For this review, take the finished solid that the model builds, in its own axes (mm). A direction names the side the tool comes from. Coordinates: 2 decimals unless noted, no trailing zeros. Loops run counter-clockwise (first coordinate to the right, second up) from the corner with the lowest first, then second, coordinate; pieces in that order, holes last. Notation, with made-up numbers: (-31.5, -39) - (-22.5, -39) arc R22 ccw to (-22.5, -25) - close; hole circle Ø1 at (12, 28). An arc over 180 degrees is marked (long way). One line per item, written item: value. Start each with the question number.
1. Take a section at D-D, the plane x = 16. State the section outline as (y, z) points, and give its area (3 significant figures).
2. Take a section at A-A, the plane y = 0. State the section outline as (x, z) points, and give its area (3 significant figures).
3. Take a section at C-C, the plane z = 0.8. State the section outline as (x, y) points, and give its area (3 significant figures).
4. Insertion check: pin 1 (1.5 mm diameter, centred on y = -10.5, z = 2, fed in from -X); pin 2 (0.6 mm diameter, centred on x = -22, z = 3.5, fed in from -Y); pin 3 (1 mm diameter, centred on y = 17.5, z = 4, fed in from +X). Each pin has a flat end and moves straight along its axis. Give the tip position at first contact, or say it passes through.
5. Take a section at B-B, the plane x = 38.25. State the section outline as (y, z) points.
6. To check wall thickness, follow line 1 (X direction, y = 26, z = 3.1); line 2 (X direction, y = -14.5, z = 2.2); line 3 (Z direction, x = 14, y = 8). State the ranges of each line that lie inside material, in increasing order. Write a range as from..to.
7. For faces 1 (the face through (0, 0, 4)), 2 (the face through (-1, 1, 0)), list the 3-axis set-ups (+Z, -Z, +X, -X, +Y, -Y) from which the entire face can be reached by the end or side of a thin tool; tool diameter is ignored.
```python
from build123d import *

# Parameters (mm, degrees)
F0_R     = 45
F0_R_2   = 1.5
F1_DEPTH = 5
F2_R     = 30
F3_DEPTH = 3
F5_DEPTH = 2


with BuildPart() as f1:
    # F0 (on Top) → F1 (new body)
    with BuildSketch(Plane.XY):
        Circle(F0_R)
        with Locations((-38.25, 0)):
            Circle(F0_R_2, mode=Mode.SUBTRACT)
        with Locations((38.25, 0)):
            Circle(F0_R_2, mode=Mode.SUBTRACT)
    extrude(amount=F1_DEPTH)

    # F2 (on face) → F3 (cut)
    with BuildSketch(Plane.XY.offset(5)):
        Circle(F2_R)
    extrude(amount=-F3_DEPTH, mode=Mode.SUBTRACT)

    # F4 (on face) → F5 (join)
    with BuildSketch(Plane.XY.offset(2)):
        with BuildLine():
            Line((-3.2170990016, 29.8270057836), (-3.2170990016, 2.8556571342))
            Line((-3.2170990016, 2.8556571342), (-29.8637777639, 2.8556571342))
            ThreePointArc((-29.8637777639, 2.8556571342), (-30, 0), (-29.8637777639, -2.8556571342))
            Line((-29.8637777639, -2.8556571342), (-3.2170990016, -2.8556571342))
            Line((-3.2170990016, -2.8556571342), (-3.2170990016, -29.8270057836))
            ThreePointArc((-3.2170990016, -29.8270057836), (0, -30), (3.2170990016, -29.8270057836))
            Line((3.2170990016, -29.8270057836), (3.2170990016, -2.8556571342))
            Line((3.2170990016, -2.8556571342), (29.8637777639, -2.8556571342))
            ThreePointArc((29.8637777639, -2.8556571342), (29.9659250893, -1.4294521823), (30, 0))
            ThreePointArc((30, 0), (29.9659250893, 1.4294521823), (29.8637777639, 2.8556571342))
            Line((29.8637777639, 2.8556571342), (3.2170990016, 2.8556571342))
            Line((3.2170990016, 2.8556571342), (3.2170990016, 29.8270057836))
            ThreePointArc((3.2170990016, 29.8270057836), (0, 30), (-3.2170990016, 29.8270057836))
        make_face()
    extrude(amount=F5_DEPTH)


solid = f1.part
```
Solutions:
1. outline: (-42.06, 0) - (42.06, 0) - (42.06, 5) - (25.38, 5) - (25.38, 2) - (2.86, 2) - (2.86, 4) - (-2.86, 4) - (-2.86, 2) - (-25.38, 2) - (-25.38, 5) - (-42.06, 5) - close
1. area: 280 mm2
2. outline: (-45, 0) - (-39.75, 0) - (-39.75, 5) - (-45, 5) - close; (-36.75, 0) - (36.75, 0) - (36.75, 5) - (30, 5) - (30, 4) - (-30, 4) - (-30, 5) - (-36.75, 5) - close; (39.75, 0) - (45, 0) - (45, 5) - (39.75, 5) - close
2. area: 360 mm2
3. outline: circle Ø90 at (0, 0); hole circle Ø3 at (-38.25, 0); hole circle Ø3 at (38.25, 0)
3. area: 6,350 mm2
4. pin 1: x = -43.93
4. pin 2: y = -39.42
4. pin 3: x = 41.67
5. outline: (-23.71, 0) - (-1.5, 0) - (-1.5, 5) - (-23.71, 5) - close; (1.5, 0) - (23.71, 0) - (23.71, 5) - (1.5, 5) - close
6. line 1: -36.73..-14.97, -3.22..3.22, 14.97..36.73
6. line 2: -42.6..-26.26, -3.22..3.22, 26.26..42.6
6. line 3: 0..2
7. face 1: +Z
7. face 2: -Z, +X, -X, +Y, -Y
